CAD build for the part. Positions are in the model's coordinates, mm. A direction names the side the tool comes from. Give positions to 0.01 mm unless a question says otherwise; leave off trailing zeros. Write each loop counter-clockwise with the first axis right and the second up, starting at its lowest first coordinate (ties: lowest second). Pieces come first, ordered by that corner, then holes. Notation, with made-up numbers: (-16, -1) -> (-7, -1) arc R24 cw to (-7, 17) -> close; hole circle Ø6 at (83.25, -9). An arc over 180 degrees is marked (long way). Answer as a JSON object with one key per item and string values.
```python
from build123d import *

# Parameters (mm, degrees)
F0_W          = 12.7
F0_H          = 12.7
F1_DEPTH      = 25.4
F1_DEPTH_BACK = 25.4
F2_DEPTH      = 25.4


with BuildPart() as f1:
    # F0 (on Right) → F1 (new body, two sides)
    with BuildSketch(Plane.YZ) as f1_sk:
        with Locations((6.35, -0.3065654278)):
            Rectangle(F0_W, F0_H)
        Polygon((0, -6.6565654278), (0, 6.0434345722), (-254, 6.0434345722), (-254, -6.6565654278), (-236.0394877579, -6.6565654278), align=None)
        Polygon((12.7, -6.6565654278), (0, -6.6565654278), (0, -242.6960531856), (0, -260.1933913213), (12.7, -260.6565654278), align=None)
        Polygon((-254, -6.6565654278), (-254, 6.0434345722), (-266.7, 6.0434345722), align=None)
        Polygon((0, -260.1933913213), (0, -242.6960531856), (-236.0394877579, -6.6565654278), (-254, -6.6565654278), (-0.4807056342, -260.1758597936), align=None)
        Polygon((12.7, -273.3565654278), (12.7, -260.6565654278), (0, -260.6565654278), align=None)
        Polygon((0, -260.6565654278), (12.7, -260.6565654278), (0, -260.1933913213), align=None)
        Polygon((0, -260.6565654278), (0, -260.1933913213), (-0.4807056342, -260.1758597936), align=None)
    extrude(amount=F1_DEPTH)
    extrude(f1_sk.sketch, amount=-F1_DEPTH_BACK)

    # F0 (on Right) → F2 (join)
    with BuildSketch(Plane.YZ):
        with Locations((6.35, -0.3065654278)):
            Rectangle(F0_W, F0_H)
        Polygon((0, -6.6565654278), (0, 6.0434345722), (-254, 6.0434345722), (-254, -6.6565654278), (-236.0394877579, -6.6565654278), align=None)
        Polygon((12.7, -6.6565654278), (0, -6.6565654278), (0, -242.6960531856), (0, -260.1933913213), (12.7, -260.6565654278), align=None)
        Polygon((-254, -6.6565654278), (-254, 6.0434345722), (-266.7, 6.0434345722), align=None)
        Polygon((0, -260.1933913213), (0, -242.6960531856), (-236.0394877579, -6.6565654278), (-254, -6.6565654278), (-0.4807056342, -260.1758597936), align=None)
        Polygon((12.7, -273.3565654278), (12.7, -260.6565654278), (0, -260.6565654278), align=None)
        Polygon((0, -260.6565654278), (12.7, -260.6565654278), (0, -260.1933913213), align=None)
        Polygon((0, -260.6565654278), (0, -260.1933913213), (-0.4807056342, -260.1758597936), align=None)
    extrude(amount=F2_DEPTH)


solid = f1.part
```
1) Mould opens along Z. For faces 1 (the flat face through (0, -120, -6.657)), 2 (the flat face through (25.4, -117, -133)), 3 (the flat face through (0, -125, 6.043)) say: released by +Z, released by -Z, zero draft, split by the parting line, or undercut.
Model answer:
{"face 1": "undercut", "face 2": "zero draft", "face 3": "released by +Z"}
2) Wall check: probe 1 along Y at (x, z) = (-16.5, -12.5); probe 2 along Z at (x, y) = (-19, -163.5); probe 3 along Z at (x, y) = (-4, -120). Give the ranges that are in metal, low to high.
Model answer:
{"probe 1": "y = -248.16 to -230.2, 0 to 12.7", "probe 2": "z = -97.16 to -79.2, -6.66 to 6.04", "probe 3": "z = -140.66 to -122.7, -6.66 to 6.04"}
3) Slice it at D-D (y = -242.5). List the corners of the cut face in (x, z), then the cut area to 3 significant figures.
Model answer:
{"outline": "(-25.4, -18.16) -> (25.4, -18.16) -> (25.4, 6.04) -> (-25.4, 6.04) -> close", "area": "1,230 mm2"}
4) 3-axis set-ups, long thin cutter, end or side, ignore diameter. For faces 4 (the flat face through (0.356, -116.367, -126.329)), 5 (the flat face through (-25.4, -117, -133)): which of +Z, -Z, +X, -X, +Y, -Y reach the whole face in a straight line?
Model answer:
{"face 4": "+X, -X", "face 5": "+Z, -Z, -X, +Y, -Y"}
5) Slice it at A-A (x = 4). List the corners of the cut face in (y, z).
Model answer:
{"outline": "(-266.7, 6.04) -> (12.7, -273.36) -> (12.7, 6.04) -> close; hole (-236.04, -6.66) -> (0, -242.7) -> (0, -6.66) -> close"}
6) Slice it at C-C (y = -160). List the corners of the cut face in (x, z), then the cut area to 3 significant figures.
Model answer:
{"outline": "(-25.4, -100.66) -> (25.4, -100.66) -> (25.4, -82.7) -> (-25.4, -82.7) -> close; (-25.4, -6.66) -> (25.4, -6.66) -> (25.4, 6.04) -> (-25.4, 6.04) -> close", "area": "1,560 mm2"}
7) Slice it at B-B (z = -208). List the corners of the cut face in (x, y).
Model answer:
{"outline": "(-25.4, -52.66) -> (25.4, -52.66) -> (25.4, -34.7) -> (-25.4, -34.7) -> close; (-25.4, 0) -> (25.4, 0) -> (25.4, 12.7) -> (-25.4, 12.7) -> close"}
8) Pin check, flat tips, straight feed: pin 1 (1 mm diameter, centred on x = -15, y = -201, fed in from -Z); pin 2 (10 mm diameter, centred on y = -44.5, z = -190, fed in from -X); pin 3 (4 mm diameter, centred on x = 4.5, y = -30, fed in from -Z). Stop position of each tip, or through.
Model answer:
{"pin 1": "stops at z = -60.16", "pin 2": "passes through", "pin 3": "stops at z = -232.66"}
